Work out the finished part from the listing and answer in its coordinate system (mm). Face numbers are marked on the shaded views. A direction names the side the tool comes from. Give positions to 0.01 mm unless a question says otherwise; leave off trailing zeros. Order: outer loops, then holes, each group sorted by start corner. A loop starts at its lowest first (then second) coordinate and runs counter-clockwise, first axis right, second up. Notation, with made-up numbers: (-30.5, -13.75) -> (-23.5, -13.75) arc R24 cw to (-23.5, -1.75) -> close; hole circle Ø4 at (-34, 53). An arc over 180 degrees is marked (long way). Answer as CSV lines item,"result". Start each with the question number.
1. A cutting plane is placed at D-D (x = 2.5). Give the vertices of the cut face in (y, z), then the cut area to 3 significant figures.
2. Find the intervals of material crossed by L1, parallel to Y at x = 0, z = 1.55; L2, parallel to X at y = -14.05, z = 4; L3, parallel to Z at x = 0.25, y = -3.75, in increasing order.
3. For the marked faces 1 and 2, determine the directions among +Z, -Z, +X, -X, +Y, -Y from which every point of the face is accessible in a straight line to the end or side of a thin tool.
4. Flat-ended cylindrical pins translate along their axes: pin 1 (2 mm diameter, centred on x = 0, y = 6, fed in from +Z); pin 2 (2.5 mm diameter, centred on x = 0, y = 9.2, fed in from -Z); pin 3 (1 mm diameter, centred on x = -2, z = 34, fed in from +Y). Find the tip coordinate at first contact, or state that the pin passes through.
5. A cutting plane is placed at A-A (x = 0). Give the vertices of the cut face in (y, z), then the cut area to 3 significant figures.
6. A cutting plane is placed at B-B (z = 4). Give the vertices of the cut face in (x, y).
7. A cutting plane is placed at C-C (y = 8.5). Give the vertices of the cut face in (x, z), then the cut area to 3 significant figures.
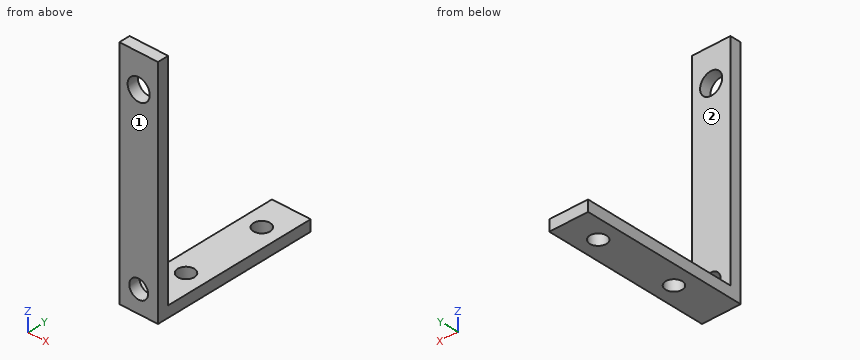
from build123d import *

# Parameters (mm, degrees)
ESBO_O2_W                = 7
ESBO_O2_H                = 30
RESSALTO_EXTRUS_O1_DEPTH = 2
ESBO_O3_W                = 7
ESBO_O3_H                = 2
RESSALTO_EXTRUS_O2_DEPTH = 40
CORTE_EXTRUS_O1_REACH    = 53.732
ESBO_O4_R                = 1.7
ESBO_O4_R_2              = 2
ESBO_O5_R                = 1.5
CORTE_EXTRUS_O2_DEPTH    = 10


with BuildPart() as part:
    # Esboço2 → Ressalto-extrusão1 (new body)
    with BuildSketch(Plane.XY):
        Rectangle(ESBO_O2_W, ESBO_O2_H)
    extrude(amount=RESSALTO_EXTRUS_O1_DEPTH)

    # Esboço3 → Ressalto-extrusão2 (add)
    with BuildSketch(Plane.XY.offset(2)):
        with Locations((0, -14)):
            Rectangle(ESBO_O3_W, ESBO_O3_H)
    extrude(amount=RESSALTO_EXTRUS_O2_DEPTH)

    # Esboço4 → Corte-extrusão1 (cut, up to next)
    with BuildSketch(Plane.XZ.offset(15), mode=Mode.PRIVATE) as corte_extrus_o1_sk1:
        with Locations(Location((0, 4, 0), (0, 0, 270))):
            Circle(ESBO_O4_R)
    corte_extrus_o1_tool1 = extrude(corte_extrus_o1_sk1.sketch, amount=-CORTE_EXTRUS_O1_REACH, mode=Mode.PRIVATE) & part.part
    # Esboço4 → Corte-extrusão1 (cut, up to next)
    with BuildSketch(Plane.XZ.offset(15), mode=Mode.PRIVATE) as corte_extrus_o1_sk2:
        with Locations(Location((0, 36, 0), (0, 0, 270))):
            Circle(ESBO_O4_R_2)
    corte_extrus_o1_tool2 = extrude(corte_extrus_o1_sk2.sketch, amount=-CORTE_EXTRUS_O1_REACH, mode=Mode.PRIVATE) & part.part
    add(corte_extrus_o1_tool1.solids().sort_by_distance((0, -15, 4))[0], mode=Mode.SUBTRACT)
    add(corte_extrus_o1_tool2.solids().sort_by_distance((0, -15, 36))[0], mode=Mode.SUBTRACT)

    # Esboço5 → Corte-extrusão2 (cut)
    with BuildSketch(Plane.XY.offset(2)):
        with Locations((0, -5.695873952)):
            Circle(ESBO_O5_R)
        with Locations((0, 9.199228267)):
            Circle(ESBO_O5_R)
    extrude(amount=-CORTE_EXTRUS_O2_DEPTH, mode=Mode.SUBTRACT)


solid = part.part
Answer sheet:
1,outline,"(-15, 0) -> (15, 0) -> (15, 2) -> (-13, 2) -> (-13, 42) -> (-15, 42) -> close"
1,area,"140 mm^2"
2,L1,"y = -15 to -7.2, -4.2 to 7.7, 10.7 to 15"
2,L2,"x = -3.5 to -1.7, 1.7 to 3.5"
2,L3,"z = 0 to 2"
3,face 1,"+Z, -Z, +X, -X, -Y"
3,face 2,"+Z, +X, -X, +Y"
4,pin 1,"stops at z = 2"
4,pin 2,"passes through"
4,pin 3,"stops at y = -13"
5,outline,"(-15, 0) -> (-7.2, 0) -> (-7.2, 2) -> (-13, 2) -> (-13, 2.3) -> (-15, 2.3) -> close; (-15, 5.7) -> (-13, 5.7) -> (-13, 34) -> (-15, 34) -> close; (-15, 38) -> (-13, 38) -> (-13, 42) -> (-15, 42) -> close; (-4.2, 0) -> (7.7, 0) -> (7.7, 2) -> (-4.2, 2) -> close; (10.7, 0) -> (15, 0) -> (15, 2) -> (10.7, 2) -> close"
5,area,"113 mm^2"
6,outline,"(-3.5, -15) -> (-1.7, -15) -> (-1.7, -13) -> (-3.5, -13) -> close; (1.7, -15) -> (3.5, -15) -> (3.5, -13) -> (1.7, -13) -> close"
7,outline,"(-3.5, 0) -> (-1.33, 0) -> (-1.33, 2) -> (-3.5, 2) -> close; (1.33, 0) -> (3.5, 0) -> (3.5, 2) -> (1.33, 2) -> close"
7,area,"8.69 mm^2"
